from build123d import *

# Parameters (mm, degrees)
SKETCH1_R            = 1.6
BOSS_EXTRUDE1_DEPTH  = 1.5
SKETCH2_W            = 1
SKETCH2_H            = 18
BOSS_EXTRUDE2_DEPTH  = 1.5
BOSS_EXTRUDE3_DEPTH  = 6
BOSS_EXTRUDE4_DEPTH  = 6
SKETCH5_W            = 1.5
SKETCH5_H            = 7
BOSS_EXTRUDE5_DEPTH  = 6
BOSS_EXTRUDE6_DEPTH  = 1.5
SKETCH7_W            = 3
SKETCH7_H            = 6
BOSS_EXTRUDE7_DEPTH  = 12
SKETCH8_W            = 3
SKETCH8_H            = 9
BOSS_EXTRUDE8_DEPTH  = 13.5
SKETCH10_W           = 3
SKETCH10_H           = 2
CUT_EXTRUDE2_DEPTH   = 141
SKETCH11_W           = 3
SKETCH11_H           = 2
BOSS_EXTRUDE9_DEPTH  = 12
SKETCH12_R           = 3.1
SKETCH12_W           = 1.5
SKETCH12_H           = 9
CUT_EXTRUDE6_DEPTH   = 86
FILLET4_R            = 4
SKETCH13_R           = 1.6
BOSS_EXTRUDE10_DEPTH = 1.5
SKETCH14_R           = 1.6
CUT_EXTRUDE7_DEPTH   = 1.5


with BuildPart() as part:
    # Sketch1 → Boss-Extrude1 (new body)
    with BuildSketch(Plane.XY):
        with BuildLine():
            Line((-35.88879481, 0), (35.88879481, 0))
            Line((35.88879481, 0), (35.88879481, 14))
            Line((35.88879481, 14), (40.88879481, 14))
            Line((40.88879481, 14), (40.88879481, -4))
            Line((40.88879481, -4), (35.88879481, -4))
            Line((35.88879481, -4), (13, -4))
            Line((13, -4), (13, -7))
            ThreePointArc((13, -7), (10, -10), (7, -7))
            Line((7, -7), (6.947208763, -7))
            Line((6.947208763, -7), (6.947208763, -4))
            Line((6.947208763, -4), (-6.947208763, -4))
            Line((-6.947208763, -4), (-6.947208763, -7))
            Line((-6.947208763, -7), (-7, -7))
            ThreePointArc((-7, -7), (-10, -10), (-13, -7))
            Line((-13, -7), (-13, -4))
            Line((-13, -4), (-35.88879481, -4))
            Line((-35.88879481, -4), (-40.88879481, -4))
            Line((-40.88879481, -4), (-40.88879481, 14))
            Line((-40.88879481, 14), (-35.88879481, 14))
            Line((-35.88879481, 14), (-35.88879481, 0))
        make_face()
        with Locations((10, -7)):
            Circle(SKETCH1_R, mode=Mode.SUBTRACT)
        with Locations((-10, -7)):
            Circle(SKETCH1_R, mode=Mode.SUBTRACT)
    extrude(amount=BOSS_EXTRUDE1_DEPTH)

    # Sketch2 → Boss-Extrude2 (add)
    with BuildSketch(Plane.XY.offset(1.5)):
        with Locations((41.38879481, 5)):
            Rectangle(SKETCH2_W, SKETCH2_H)
        with Locations((-41.38879481, 5)):
            Rectangle(SKETCH2_W, SKETCH2_H)
    extrude(amount=-BOSS_EXTRUDE2_DEPTH)

    # Sketch3 → Boss-Extrude3 (add)
    with BuildSketch(Plane.XY.offset(1.5)):
        Polygon((35.88879481, 14), (41.88879481, 14), (41.88879481, 4), (41.38879481, 4), (41.38879481, 13.5), (36.68879481, 13.5), (36.68879481, 13), (35.88879481, 13), align=None)
        Polygon((-36.68879481, 13.5), (-41.38879481, 13.5), (-41.38879481, 4), (-41.88879481, 4), (-41.88879481, 14), (-35.88879481, 14), (-35.88879481, 13), (-36.68879481, 13), align=None)
    extrude(amount=BOSS_EXTRUDE3_DEPTH)

    # Sketch4 → Boss-Extrude4 (add)
    with BuildSketch(Plane.XY.offset(7.5)):
        Polygon((-41.38879481, 4), (-41.13879481, 4), (-41.13879481, 13.12888012), (-41.13879481, 13.25), (-36.68879481, 13.25), (-36.68879481, 13.5), (-41.38879481, 13.5), align=None)
        Polygon((41.38879481, 13.5), (41.38879481, 4), (41.13879481, 4), (41.13879481, 13.12888012), (41.13879481, 13.25), (36.68879481, 13.25), (36.68879481, 13.5), align=None)
    extrude(amount=-BOSS_EXTRUDE4_DEPTH)

    # Sketch5 → Boss-Extrude5 (add)
    with BuildSketch(Plane.XY.offset(1.5)):
        with Locations((-36.63879481, 3.5)):
            Rectangle(SKETCH5_W, SKETCH5_H)
        with Locations((36.63879481, 3.5)):
            Rectangle(SKETCH5_W, SKETCH5_H)
    extrude(amount=BOSS_EXTRUDE5_DEPTH)

    # Sketch6 → Boss-Extrude6 (add)
    with BuildSketch(Plane.XY.offset(1.5)):
        Polygon((41.88879481, -4), (41.88879481, -6), (29.88879481, -6), (27.88879481, -4), align=None)
        Polygon((-27.88879481, -4), (-41.88879481, -4), (-41.88879481, -6), (-29.88879481, -6), align=None)
    extrude(amount=-BOSS_EXTRUDE6_DEPTH)

    # Sketch7 → Boss-Extrude7 (add)
    with BuildSketch(Plane.XY.offset(1.5)):
        with Locations((37.38879481, -3)):
            Rectangle(SKETCH7_W, SKETCH7_H)
        with Locations((-37.38879481, -3)):
            Rectangle(SKETCH7_W, SKETCH7_H)
    extrude(amount=BOSS_EXTRUDE7_DEPTH)

    # Sketch8 → Boss-Extrude8 (add)
    with BuildSketch(Plane.XY.offset(13.5)):
        with Locations((-37.38879481, -4.5)):
            Rectangle(SKETCH8_W, SKETCH8_H)
        with Locations((37.38879481, -4.5)):
            Rectangle(SKETCH8_W, SKETCH8_H)
    extrude(amount=-BOSS_EXTRUDE8_DEPTH)

    # Sketch10 → Cut-Extrude2 (cut)
    with BuildSketch(Plane.XY.offset(13.5)):
        with Locations((-37.38879481, -8)):
            Rectangle(SKETCH10_W, SKETCH10_H)
        with Locations((37.38879481, -8)):
            Rectangle(SKETCH10_W, SKETCH10_H)
    extrude(amount=-CUT_EXTRUDE2_DEPTH, mode=Mode.SUBTRACT)

    # Sketch11 → Boss-Extrude9 (add)
    with BuildSketch(Plane.XY.offset(13.5)):
        with Locations((-37.38879481, 1)):
            Rectangle(SKETCH11_W, SKETCH11_H)
        with Locations((37.38879481, 1)):
            Rectangle(SKETCH11_W, SKETCH11_H)
    extrude(amount=-BOSS_EXTRUDE9_DEPTH)

    # Sketch12 → Cut-Extrude6 (cut)
    with BuildSketch(Plane(origin=(38.88879481, 0, 0), x_dir=(0, 0, -1), z_dir=(1, 0, 0))):
        with Locations((-7.5, -2.5)):
            Circle(SKETCH12_R)
        with Locations((-12.75, -2.5)):
            Rectangle(SKETCH12_W, SKETCH12_H)
    extrude(amount=-CUT_EXTRUDE6_DEPTH, mode=Mode.SUBTRACT)

    # Fillet4
    fillet4_edges = [part.edges().sort_by_distance(p)[0] for p in [
        (37.38879481, 2, 12),
        (37.38879481, -7, 12),
        (-37.38879481, -7, 12),
        (-37.38879481, 2, 12),
    ]]
    fillet(fillet4_edges, radius=FILLET4_R)

    # Sketch13 → Boss-Extrude10 (add)
    with BuildSketch(Plane.XY.offset(1.5)):
        with BuildLine():
            Line((-29, -7), (-29, -2.59629788))
            Line((-29, -2.59629788), (-35, -2.59629788))
            Line((-35, -2.59629788), (-35, -7))
            ThreePointArc((-35, -7), (-32, -10), (-29, -7))
        make_face()
        with Locations((-32, -7)):
            Circle(SKETCH13_R, mode=Mode.SUBTRACT)
        with BuildLine():
            Line((35, -2.59629788), (29, -2.59629788))
            Line((29, -2.59629788), (29, -7))
            ThreePointArc((29, -7), (32, -10), (35, -7))
            Line((35, -7), (35, -2.59629788))
        make_face()
        with Locations((32, -7)):
            Circle(SKETCH13_R, mode=Mode.SUBTRACT)
    extrude(amount=-BOSS_EXTRUDE10_DEPTH)

    # Sketch14 → Cut-Extrude7 (cut)
    with BuildSketch(Plane.XY.offset(1.5)):
        with Locations((-32, -7)):
            Circle(SKETCH14_R)
        with Locations((32, -7)):
            Circle(SKETCH14_R)
    extrude(amount=-CUT_EXTRUDE7_DEPTH, mode=Mode.SUBTRACT)


solid = part.part
Geometry: final body of the model. Coordinates: model frame, mm. A direction names the side the tool comes from. Coordinates: 2 decimals unless noted, no trailing zeros. Order: outer loops, then holes, each group sorted by start corner. A loop starts at its lowest first (then second) coordinate and runs counter-clockwise, first axis right, second up. Notation, with made-up numbers: M 8.5,18.5 L 59.5,18.5 A19 cw 59.5,40.5 Z; hole C -8.75,82.5 d11. An arc over 180 degrees is marked long. One line per question, with ' | ' between items. Start each with the question number.
Item 1: Draft query along Z for faces 1 (the cylindrical face through (37.4, -2.4, 10.6)), 2 (the cylindrical face through (-32, -10, 1)), 3 (the flat face through (-0.5, -3.8, 1.5)). Return one class per face: released by +Z, released by -Z, zero draft, split by the parting line, or undercut.
Item 2: Cut plane C-C, the plane x = -1. Return the cut outline in (y, z).
Item 3: Set-up query: faces 4 (the flat face through (-40, -6, 1)), 5 (the cylindrical face through (-11.27, -7.97, 0.74)), 6 (the flat face through (39, 13.25, 5)), 7 (the flat face through (-20, -4, 1)), 8 (the flat face through (-41.3, 10.9, 7.5)). Return all of +Z, -Z, +X, -X, +Y, -Y with unobstructed straight access to the full face (end or side cutting, diameter ignored); none if empty.
Item 4: Cut plane A-A, the plane x = 32. Return the cut outline in (y, z), then the cut area to 3 significant figures.
Item 5: Pin query (flat end, axial travel): pin 1 Ø1.6 at (x, z) = (-2, 0.5) entering from +Y; pin 2 Ø0.8 at (x, z) = (41.5, 5.5) entering from -Y; pin 3 Ø1.2 at (x, z) = (40, 0.5) entering from -Y. Return the tip coordinate at first contact, or that it passes through.
Item 6: Cut plane B-B, the plane z = 6. Count the separate pieces of the cut face and the enclosed holes in it, then the cut area to 3 significant figures.
Item 7: Ray query, probe 1 along X at (y, z) = (8.5, 2); probe 2 along X at (y, z) = (3.75, 3.5); probe 3 along Y at (x, z) = (32, 0.7). Return the intervals inside material, ascending. Write a range as [from, to].
A:
1) face 1: undercut | face 2: zero draft | face 3: released by +Z
2) outline: M -4,0 L 0,0 L 0,1.5 L -4,1.5 Z
3) face 4: +Z, -Z, -X, -Y | face 5: +Z, -Z | face 6: +Z | face 7: +Z, -Z, -Y | face 8: +Z, +X, -X, +Y
4) outline: M -10,0 L -8.6,0 L -8.6,1.5 L -10,1.5 Z; M -5.4,0 L 0,0 L 0,1.5 L -5.4,1.5 Z | area: 10.2 mm2
5) pin 1: stops at y = 0 | pin 2: stops at y = 4 | pin 3: stops at y = -6
6) separate pieces: 6 | enclosed holes: 0 | area: 59.7 mm2
7) probe 1: x = [-41.89, -41.14], [41.14, 41.89] | probe 2: x = [-37.39, -35.89], [35.89, 37.39] | probe 3: y = [-10, -8.6], [-5.4, 0]
